Model file for the job. Use its own axes, mm. Face numbers are marked on the shaded views. A direction names the side the tool comes from. Coordinates: 2 decimals unless noted, no trailing zeros. Write each loop counter-clockwise with the first axis right and the second up, starting at its lowest first coordinate (ties: lowest second). Pieces come first, ordered by that corner, then holes. Notation, with made-up numbers: (69.25, 37) - (109.25, 37) arc R15 cw to (109.25, 43) - close; hole circle Ø10 at (47, 14). An arc over 180 degrees is marked (long way). Put each result on its own line as item: value. Start each with the question number.
1. Saw through at A-A, the plane x = 0. Write the cut outline in (y, z).
2. Saw through at C-C, the plane z = 11.5. Write the cut outline in (x, y).
3. Drop flat-ended pins along their axis: P1, Ø0.8, axis at x = 2, z = 14, coming from the +Y side; P2, Ø4, axis at x = 1.5, y = -3.5, coming from the -Z side; P3, Ø1.5, axis at x = 0.5, y = 7.5, coming from the +Z side; P4, Ø1, axis at x = 5.5, y = 6, coming from the +Z side. Give the stop position or say it passes through.
4. Drill centre lines: L1, parallel to Z at x = 0, y = -4.25; L2, parallel to X at y = -6, z = 11; L3, parallel to X at y = 7, z = 11.65. Where is each one in solid material? Low to high. Write a range as from..to.
5. Saw through at D-D, the plane x = 8.5. Write the cut outline in (y, z), plus the area to 4 significant figures.
6. Which spindle directions (+Z, -Z, +X, -X, +Y, -Y) get a long thin tool onto all of the face, cutting with end or side? Do the marked faces 1 and 2. Say none if no direction does.
7. Pull direction X, two halves, no side cores. Call the marked faces 3, 4, 5 and 6: released by +X, released by -X, zero draft, split by the parting line, or undercut.
8. Saw through at B-B, the plane y = 7. Write the cut outline in (x, z), plus the area to 3 significant figures.
```python
from build123d import *

# Parameters (mm, degrees)
F0_W     = 20
F0_H     = 20
F1_DEPTH = 15
F2_W     = 50.179663
F2_H     = 15.178498
F3_DEPTH = 1.5
F4_R     = 2.5
F5_DEPTH = 4
F6_R     = 1
F7_DEPTH = 25


with BuildPart() as f1:
    # F0 (on Top) → F1 (new body)
    with BuildSketch(Plane.XY):
        Rectangle(F0_W, F0_H)
    extrude(amount=F1_DEPTH)

    # F2 (on face) → F3 (cut)
    with BuildSketch(Plane.XY.offset(15)):
        with Locations((-0.497311, 12.589249)):
            Rectangle(F2_W, F2_H)
    extrude(amount=-F3_DEPTH, mode=Mode.SUBTRACT)

    # F4 (on face) → F5 (cut)
    with BuildSketch(Plane.XY.offset(13.5)):
        with Locations((0, 7)):
            Circle(F4_R)
    extrude(amount=-F5_DEPTH, mode=Mode.SUBTRACT)

    # F6 (on face) → F7 (cut)
    with BuildSketch(Plane(origin=(0, 5, 0), x_dir=(-1, 0, 0), z_dir=(0, 1, 0))):
        with Locations((0, 11)):
            Circle(F6_R)
    extrude(amount=-F7_DEPTH, mode=Mode.SUBTRACT)


solid = f1.part
```
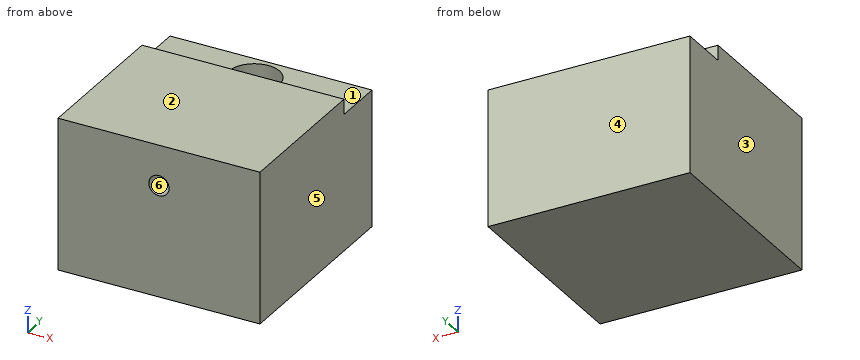
Final values:
1. outline: (-10, 0) - (10, 0) - (10, 13.5) - (9.5, 13.5) - (9.5, 9.5) - (4.5, 9.5) - (4.5, 10) - (-10, 10) - close; (-10, 12) - (4.5, 12) - (4.5, 13.5) - (5, 13.5) - (5, 15) - (-10, 15) - close
2. outline: (-10, -10) - (-0.87, -10) - (-0.87, 4.65) arc R2.5 cw (long way) to (0.87, 4.65) - (0.87, -10) - (10, -10) - (10, 10) - (-10, 10) - close
3. P1: stops at y = 5
3. P2: stops at z = 0
3. P3: stops at z = 9.5
3. P4: stops at z = 13.5
4. L1: z = 0..10, 12..15
4. L2: x = -10..-1, 1..10
4. L3: x = -10..-2.5, 2.5..10
5. outline: (-10, 0) - (10, 0) - (10, 13.5) - (5, 13.5) - (5, 15) - (-10, 15) - close
5. area: 292.5 mm²
6. face 1: +Z, +X, -X, +Y
6. face 2: +Z, +X, -X, +Y, -Y
7. face 3: released by -X
7. face 4: zero draft
7. face 5: released by +X
7. face 6: undercut
8. outline: (-10, 0) - (10, 0) - (10, 13.5) - (2.5, 13.5) - (2.5, 9.5) - (-2.5, 9.5) - (-2.5, 13.5) - (-10, 13.5) - close
8. area: 250 mm²
